Part model, mm, in its own coordinate system. A direction names the side the tool comes from. Round coordinates to 2 decimals unless told otherwise and drop trailing zeros. Write each loop counter-clockwise with the first axis right and the second up, starting at its lowest first coordinate (ties: lowest second). Pieces come first, ordered by that corner, then holes. Notation, with made-up numbers: (32.25, 63.25) -> (50.25, 63.25) arc R9 ccw to (50.25, 76.25) -> close; hole circle Ø6 at (-24, 48.25). An arc over 180 degrees is marked (long way). Return JSON: item names as keys, results as strings. Group by question number.
(1) Saw through at A-A (x = -1.5). List the corners of the cut face in (y, z), plus the area to 3 significant figures.
(2) Saw through at C-C (z = 3.9). List the corners of the cut face in (x, y), plus the area to 3 significant figures.
(3) Mould opens along X. For faces 4 (the flat face through (55, 47, 2)), 5 (the cylindrical face through (110.35, 25.59, 2.37)), 6 (the flat face through (-30.489, 77, 2)), 7 (the flat face through (100, 0, 2)) say: +X half, -X half, draft (parallel to the pull), parting line (faces both ways), or undercut.
(4) Saw through at D-D (y = 49). List the corners of the cut face in (x, z).
(5) Saw through at B-B (y = 85). List the corners of the cut face in (x, z), plus the area to 3 significant figures.
(6) Drill centre lines: L1, parallel to Y at x = -13.5, z = 0.4; L2, parallel to X at y = 70, z = 0.2; L3, parallel to X at y = 87.5, z = 2.6. Where is each one in solid material? Low to high. Write a range as from..to.
(7) Drop flat-ended pins along their axis: pin 1 Ø1.4 at (x, z) = (-79.5, 1.5) entering from -Y; pin 2 Ø1.4 at (x, z) = (124.5, 3) entering from -Y. Give the stop position or say it passes through.
(8) Tool access for faces 1 (the flat face through (133, 36.4, 2)), 2 (the flat face through (-73, 60, 2)), 3 (the flat face through (107.5, 9, 2)): list every direction of +Z, -Z, +X, -X, +Y, -Y with a clear straight run to the whole face (end or side of a thin tool).
from build123d import *

# Parameters (mm, degrees)
SALIENTE_EXTRUIR2_DEPTH = 4.8


with BuildPart() as part:
    # Croquis1 → Saliente-Extruir2 (new body)
    with BuildSketch(Plane.XY):
        with BuildLine():
            Line((-17.5, 0), (17.5, 0))
            ThreePointArc((17.5, 0), (55, 25.580282757), (92.5, 0))
            Line((92.5, 0), (107.5, 0))
            Line((107.5, 0), (107.5, 18.6))
            ThreePointArc((107.5, 18.6), (110.428932188, 25.671067812), (117.5, 28.6))
            Line((117.5, 28.6), (137.513068614, 28.6))
            Line((137.513068614, 28.6), (137.513068614, 36.4))
            Line((137.513068614, 36.4), (127.513068614, 36.4))
            Line((127.513068614, 36.4), (59.018966471, 60.165688958))
            Line((59.018966471, 60.165688958), (25.594010768, 100))
            Line((25.594010768, 100), (-104.405989232, 100))
            Line((-104.405989232, 100), (-127.5, 60))
            Line((-127.5, 60), (-127.5, 0))
            Line((-127.5, 0), (-92.5, 0))
            ThreePointArc((-92.5, 0), (-55, 26.176046527), (-17.5, 0))
        make_face()
        Polygon((-116.916975087, 60), (-98.205737613, 92.999006125), (-30.488878185, 92.999006125), (-30.488878185, 60), align=None, mode=Mode.SUBTRACT)
        with BuildLine():
            Line((-17.5, 92.999006125), (-17.5, 14.847400468))
            Line((-17.5, 14.847400468), (14.466697892, 14.847400468))
            ThreePointArc((14.466697892, 14.847400468), (31.548577024, 31.595792779), (55, 36.321255728))
            Line((55, 36.321255728), (55, 58.860748488))
            Line((55, 58.860748488), (24.578803898, 92.999006125))
            Line((24.578803898, 92.999006125), (-17.5, 92.999006125))
        make_face(mode=Mode.SUBTRACT)
    extrude(amount=SALIENTE_EXTRUIR2_DEPTH)


solid = part.part
Computed values:
{
 "1": {"outline": "(0, 0) -> (14.85, 0) -> (14.85, 4.8) -> (0, 4.8) -> close; (93, 0) -> (100, 0) -> (100, 4.8) -> (93, 4.8) -> close", "area": "105 mm2"},
 "2": {"outline": "(-127.5, 0) -> (-92.5, 0) arc R39.95 cw to (-17.5, 0) -> (17.5, 0) arc R40.28 cw to (92.5, 0) -> (107.5, 0) -> (107.5, 18.6) arc R10 cw to (117.5, 28.6) -> (137.51, 28.6) -> (137.51, 36.4) -> (127.51, 36.4) -> (59.02, 60.17) -> (25.59, 100) -> (-104.41, 100) -> (-127.5, 60) -> close; hole (-116.92, 60) -> (-30.49, 60) -> (-30.49, 93) -> (-98.21, 93) -> close; hole (-17.5, 14.85) -> (14.47, 14.85) arc R42.06 cw to (55, 36.32) -> (55, 58.86) -> (24.58, 93) -> (-17.5, 93) -> close", "area": "10,500 mm2"},
 "3": {"face 4": "undercut", "face 5": "+X half", "face 6": "undercut", "face 7": "draft"},
 "4": {"outline": "(-127.5, 0) -> (-17.5, 0) -> (-17.5, 4.8) -> (-127.5, 4.8) -> close; (55, 0) -> (91.2, 0) -> (91.2, 4.8) -> (55, 4.8) -> close"},
 "5": {"outline": "(-113.07, 0) -> (-102.74, 0) -> (-102.74, 4.8) -> (-113.07, 4.8) -> close; (-30.49, 0) -> (-17.5, 0) -> (-17.5, 4.8) -> (-30.49, 4.8) -> close; (31.71, 0) -> (38.18, 0) -> (38.18, 4.8) -> (31.71, 4.8) -> close", "area": "143 mm2"},
 "6": {"L1": "0..14.85, 93..100", "L2": "-121.73..-111.25, -30.49..-17.5, 45.07..50.77", "L3": "-111.62..-101.32, -30.49..-17.5, 29.48..36.08"},
 "7": {"pin 1": "y = 17.23", "pin 2": "y = 28.6"},
 "8": {"face 1": "+Z, -Z, +X, +Y", "face 2": "+Z, -Z", "face 3": "+Z, -Z, +X, -Y"}
}
